Here's how the part is built. I have some questions about the finished solid (model axes, mm). Round coordinates to 2 decimals unless told otherwise and drop trailing zeros. Loops run counter-clockwise (first coordinate to the right, second up) from the corner with the lowest first, then second, coordinate; pieces in that order, holes last. Notation, with made-up numbers: M 83.5,-4.5 L 88.5,-4.5 A24 cw 88.5,6.5 Z; hole C 69,8.5 d10. An arc over 180 degrees is marked long. Use a Markdown table: item, result.
```python
from build123d import *

# Parameters (mm, degrees)
SKETCH1_R           = 2
SKETCH1_R_2         = 12.625986588
BOSS_EXTRUDE1_DEPTH = 6
SKETCH2_R           = 2
CUT_EXTRUDE1_DEPTH  = 10


with BuildPart() as part:
    # Sketch1 → Boss-Extrude1 (new body)
    with BuildSketch(Plane.XY):
        Polygon((20, -60), (60, -20), (60, 0), (0, 0), (-60, 0), (-60, -60), (0, -60), align=None)
        with Locations((50, -10)):
            Circle(SKETCH1_R, mode=Mode.SUBTRACT)
        with Locations((30, -10)):
            Circle(SKETCH1_R, mode=Mode.SUBTRACT)
        with Locations((10, -50)):
            Circle(SKETCH1_R, mode=Mode.SUBTRACT)
        with Locations((10, -30)):
            Circle(SKETCH1_R, mode=Mode.SUBTRACT)
        with Locations((-33.365647648, -24.93)):
            Circle(SKETCH1_R_2, mode=Mode.SUBTRACT)
    extrude(amount=BOSS_EXTRUDE1_DEPTH)

    # Sketch2 → Cut-Extrude1 (cut)
    with BuildSketch(Plane(origin=(0, 0, 0), x_dir=(-1, 0, 0), z_dir=(0, 0, -1))):
        with Locations((17.915647648, -9.48)):
            Circle(SKETCH2_R)
        with Locations((17.915647648, -40.43)):
            Circle(SKETCH2_R)
        with Locations((48.865647648, -9.48)):
            Circle(SKETCH2_R)
        with Locations((48.865647648, -40.43)):
            Circle(SKETCH2_R)
    extrude(amount=-CUT_EXTRUDE1_DEPTH, mode=Mode.SUBTRACT)


solid = part.part
```
Q1. Imagine slicing it at C-C, the plane z = 2.7. Give the number of separate pieces and of enclosed holes in the cut face, then the cut area to 3 significant figures.
Return value:
| item | result |
|---|---|
| separate pieces | 1 |
| enclosed holes | 9 |
| area | 5,800 mm^2 |
Q2. I need wall thicknesses on line 1 (Y direction, x = 10, z = 3.75); line 2 (X direction, y = -11, z = 1.9); line 3 (Y direction, x = -30, z = 0.6). Which ranges of each line are inside material? Lowest first, please. Write a range as from..to.
Return value:
| item | result |
|---|---|
| line 1 | y = -60..-52, -48..-32, -28..0 |
| line 2 | x = -60..-50.17, -47.57..-19.22, -16.62..28.27, 31.73..48.27, 51.73..60 |
| line 3 | y = -60..-37.1, -12.76..0 |
Q3. Imagine slicing it at D-D, the plane x = 30. Please give me the cut outline in (y, z).
Return value:
| item | result |
|---|---|
| outline | M -50,0 L -12,0 L -12,6 L -50,6 Z; M -8,0 L 0,0 L 0,6 L -8,6 Z |
Q4. Imagine slicing it at A-A, the plane y = -50. Please give me the cut outline in (x, z), then the cut area to 3 significant figures.
Return value:
| item | result |
|---|---|
| outline | M -60,0 L 8,0 L 8,6 L -60,6 Z; M 12,0 L 30,0 L 30,6 L 12,6 Z |
| area | 516 mm^2 |
Q5. We'd pull the mould along Y, two halves only. Please class faces 1 (the cylindrical face through (-16.33, -10.7, 2.96)), 2 (the flat face through (40, -40, 3)), 3 (the flat face through (-60, -30, 3)): pulls with the +Y half, pulls with the -Y half, needs draft (parallel to the pull), parting line crosses it, or undercut.
Return value:
| item | result |
|---|---|
| face 1 | undercut |
| face 2 | pulls with the -Y half |
| face 3 | needs draft |
Q6. Imagine slicing it at B-B, the plane x = 10. Please give me the cut outline in (y, z).
Return value:
| item | result |
|---|---|
| outline | M -60,0 L -52,0 L -52,6 L -60,6 Z; M -48,0 L -32,0 L -32,6 L -48,6 Z; M -28,0 L 0,0 L 0,6 L -28,6 Z |
Q7. Will these pins go through, and if not, where does the flat tip stop? P1, Ø3, axis at x = -17.92, y = -9.48, coming from the -Z side; P2, Ø3, axis at x = 39.5, z = 3, coming from the -Y side; P3, Ø3, axis at y = -39.5, z = 3, coming from the +X side.
Return value:
| item | result |
|---|---|
| P1 | passes through |
| P2 | stops at y = -42 |
| P3 | stops at x = 42 |
